Source: three-view drawing plus pictorial views. Frame: mm from the lowest corner of the part. A direction names the side the tool comes from. Coordinates: 2 decimals unless noted, no trailing zeros. Write each loop counter-clockwise with the first axis right and the second up, starting at its lowest first coordinate (ties: lowest second). Pieces come first, ordered by that corner, then holes. Notation, with made-up numbers: (71, 36.5) - (109, 36.5) arc R19 cw to (109, 43.5) - close; hole circle Ø4 at (-25, 62). An arc over 180 degrees is marked (long way). Put each result on its own line as item: value. Start each with the question number.
1. Pin query (flat end, axial travel): pin 1 (3.5 mm diameter, centred on y = 29, z = 20.5, fed in from +X); pin 2 (1 mm diameter, centred on x = 16.5, y = 23, fed in from +Z). Return the tip coordinate at first contact, or that it passes through.
2. Cut plane A-A, the plane z = 7.9. Return loops of the section in (x, y) (3 decimals).
3. Cut plane B-B, the plane x = 20.25. Return loops of the section in (y, z) (3 decimals).
4. Cut plane C-C, the plane y = 47.5. Return loops of the section in (x, z).
5. Cut plane D-D, the plane z = 19.05. Return loops of the section in (x, y) (3 decimals), and give its area (3 significant figures).
6. Access query for the marked faces 1 and 2. Directions: +Z, -Z, +X, -X, +Y, -Y. A direction counts if a zero-diameter tool reaches every point of the face in a straight line with its end or side. Return the directions, or none.
7. Line query: line 1 (X direction, y = 44.5, z = 7.25); line 2 (Y direction, x = 20.25, z = 8) (3 decimals); line 3 (X direction, y = 49.5, z = 7.9). Output: solid intervals per line, ascending.
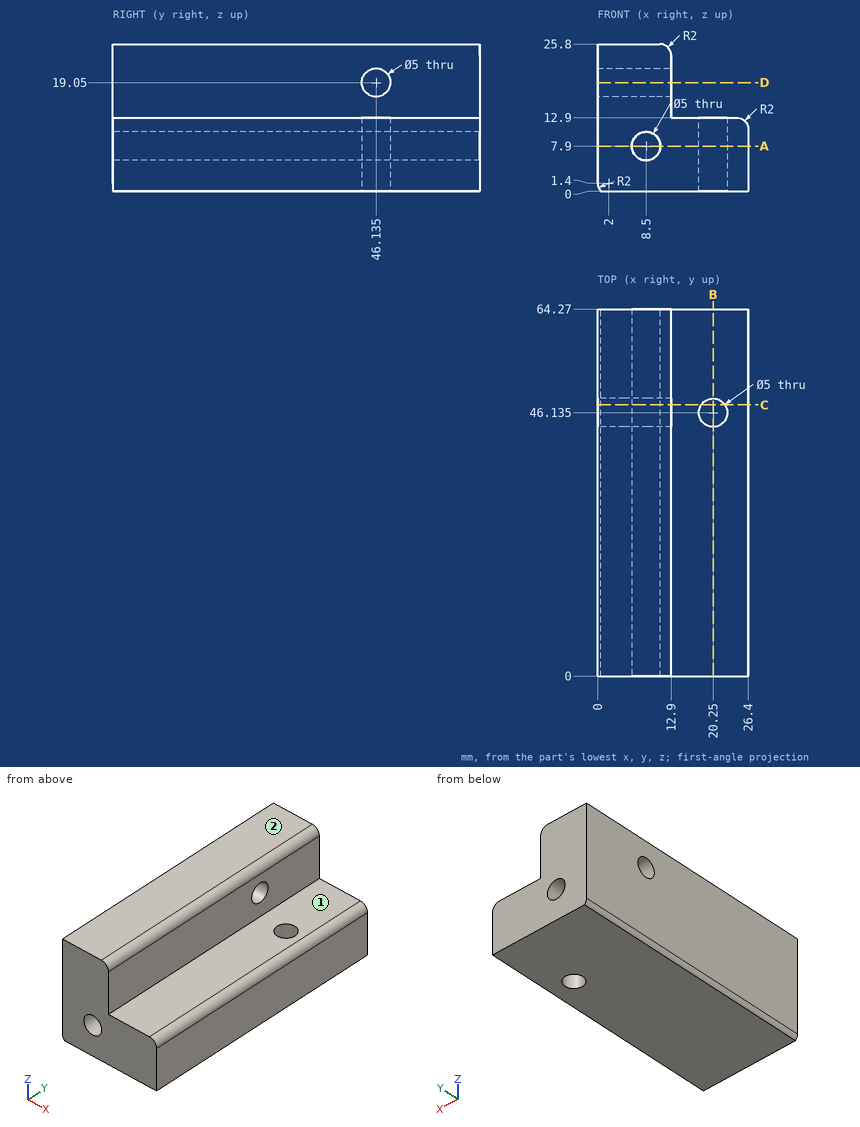
Report:
1. pin 1: stops at x = 12.9
1. pin 2: stops at z = 12.9
2. outline: (0, 0) - (6, 0) - (6, 64.27) - (0, 64.27) - close; (11, 0) - (26.4, 0) - (26.4, 64.27) - (11, 64.27) - close; hole circle Ø5 at (20.25, 46.135)
3. outline: (0, 0) - (43.635, 0) - (43.635, 12.9) - (0, 12.9) - close; (48.635, 0) - (64.27, 0) - (64.27, 12.9) - (48.635, 12.9) - close
4. outline: (0, 1.4) arc R2 ccw to (0.57, 0) - (18.16, 0) - (18.16, 12.9) - (12.9, 12.9) - (12.9, 16.96) - (0, 16.96) - close; (0, 21.14) - (12.9, 21.14) - (12.9, 23.8) arc R2 ccw to (10.9, 25.8) - (0, 25.8) - close; (22.34, 0) - (26.4, 0) - (26.4, 10.9) arc R2 ccw to (24.4, 12.9) - (22.34, 12.9) - close; hole circle Ø5 at (8.5, 7.9)
5. outline: (0, 0) - (12.9, 0) - (12.9, 43.635) - (0, 43.635) - close; (0, 48.635) - (12.9, 48.635) - (12.9, 64.27) - (0, 64.27) - close
5. area: 765 mm^2
6. face 1: +Z, +X, +Y, -Y
6. face 2: +Z, +X, -X, +Y, -Y
7. line 1: x = 0 to 6.09, 10.91 to 18.36, 22.14 to 26.4
7. line 2: y = 0 to 43.635, 48.635 to 64.27
7. line 3: x = 0 to 6, 11 to 26.4
